Here's how the part is built. I have some questions about the finished solid (model axes, mm). Face numbers are marked on the shaded views. Coordinates: 2 decimals unless noted, no trailing zeros. Write each loop counter-clockwise with the first axis right and the second up, starting at its lowest first coordinate (ties: lowest second). Pieces come first, ordered by that corner, then holes.
Autodesk Inventor part; units mm, degrees
ref_plane "YZ Plane" through (0, 0, 0) normal (1, 0, 0) x (0, 1, 0)
ref_plane "XZ Plane" through (0, 0, 0) normal (0, 1, 0) x (-1, 0, 0)
ref_plane "XY Plane" through (0, 0, 0) normal (0, 0, 1) x (1, 0, 0)
sketch "Sketch1" plane through (0, 0, 0) normal (0, 0, 1) x (1, 0, 0)
  circle A0 centre (0, 0) radius 52.75
  dimension "d0" = 105.5
extrude "Extrusion1" add sketch "Sketch1" along normal blind 7
fillet "Fillet1" radius 4 1 edges at (-52.75, 0, 7)
sketch "Sketch2" plane through (0, 0, 0) normal (0, 0, -1) x (-1, 0, 0)
  circle A0 centre (0, 0) radius 51.8
  circle A1 centre (0, 0) radius 52.75
  circle A2 centre (0, 0) radius 52.75
  dimension "d4" = 103.6
  dimension "d69" = 0
extrude "Extrusion2" cut sketch "Sketch2" against normal blind 3
sketch "Sketch3" plane through (0, 0, 0) normal (0, 0, -1) x (-1, 0, 0)
  circle A0 centre (0, 0) radius 48.75
extrude "Extrusion3" cut sketch "Sketch3" against normal blind 6
sketch "Sketch6" plane through (0, 0, 7) normal (0, 0, 1) x (1, 0, 0)
  circle A0 centre (0, 0) radius 15 construction
  circle A1 centre (15, 0) radius 1
  circle A2 centre (14.0954, 5.1303) radius 1
  circle A3 centre (11.4907, 9.6418) radius 1
  circle A4 centre (7.5, 12.9904) radius 1
  circle A5 centre (2.6047, 14.7721) radius 1
  circle A6 centre (-2.6047, 14.7721) radius 1
  circle A7 centre (-7.5, 12.9904) radius 1
  circle A8 centre (-11.4907, 9.6418) radius 1
  circle A9 centre (-14.0954, 5.1303) radius 1
  circle A10 centre (-15, 0) radius 1
  circle A11 centre (-14.0954, -5.1303) radius 1
  circle A12 centre (-11.4907, -9.6418) radius 1
  circle A13 centre (-7.5, -12.9904) radius 1
  circle A14 centre (-2.6047, -14.7721) radius 1
  circle A15 centre (2.6047, -14.7721) radius 1
  circle A16 centre (7.5, -12.9904) radius 1
  circle A17 centre (11.4907, -9.6418) radius 1
  circle A18 centre (14.0954, -5.1303) radius 1
  circle A19 centre (0, 0) radius 10 construction
  circle A20 centre (0, -10) radius 1
  circle A21 centre (4.3388, -9.0097) radius 1
  circle A22 centre (7.8183, -6.2349) radius 1
  circle A23 centre (9.7493, -2.2252) radius 1
  circle A24 centre (9.7493, 2.2252) radius 1
  circle A25 centre (7.8183, 6.2349) radius 1
  circle A26 centre (4.3388, 9.0097) radius 1
  circle A27 centre (0, 10) radius 1
  circle A28 centre (-4.3388, 9.0097) radius 1
  circle A29 centre (-7.8183, 6.2349) radius 1
  circle A30 centre (-9.7493, 2.2252) radius 1
  circle A31 centre (-9.7493, -2.2252) radius 1
  circle A32 centre (-7.8183, -6.2349) radius 1
  circle A33 centre (-4.3388, -9.0097) radius 1
  circle A34 centre (0, 0) radius 5 construction
  circle A35 centre (0, -5) radius 1
  circle A36 centre (4.3301, -2.5) radius 1
  circle A37 centre (4.3301, 2.5) radius 1
  circle A38 centre (0, 5) radius 1
  circle A39 centre (-4.3301, 2.5) radius 1
  circle A40 centre (-4.3301, -2.5) radius 1
  dimension "d44" = 30
  dimension "d50" = 20
  dimension "d56" = 10
  dimension "d45" = 2
  dimension "d48" = 360
  dimension "d51" = 2
  dimension "d54" = 360
  dimension "d57" = 2
  dimension "d60" = 360
hole "Hole1" at (0, 5, 7) at (0, 10, 7) at (4.3388, 9.0097, 7) at (7.8183, 6.2349, 7) at (7.5, 12.9904, 7) at (4.3301, 2.5, 7) at (9.7493, 2.2252, 7) at (0, 0, 7) at (0, 0, 7) at (0, 0, 7) at (4.3301, -2.5, 7) at (-7.8183, 6.2349, 7) at (-4.3301, -2.5, 7) at (0, -5, 7) at (0, 0, 7) at (15, 0, 7) at (14.0954, 5.1303, 7) at (11.4907, 9.6418, 7) at (2.6047, 14.7721, 7) at (-4.3388, 9.0097, 7) at (-11.4907, 9.6418, 7) at (-7.5, 12.9904, 7) at (-2.6047, 14.7721, 7) at (11.4907, -9.6418, 7) at (9.7493, -2.2252, 7) at (7.8183, -6.2349, 7) at (14.0954, -5.1303, 7) at (-14.0954, 5.1303, 7) at (-15, 0, 7) at (-14.0954, -5.1303, 7) at (-11.4907, -9.6418, 7) at (-7.5, -12.9904, 7) at (-4.3301, 2.5, 7) at (-4.3388, -9.0097, 7) at (-7.8183, -6.2349, 7) at (-9.7493, 2.2252, 7) at (-9.7493, -2.2252, 7) at (-2.6047, -14.7721, 7) at (2.6047, -14.7721, 7) at (7.5, -12.9904, 7) at (4.3388, -9.0097, 7) at (0, -10, 7) direction (0, 0, -1) diameter 1.778 depth 10.688
fillet "Fillet2" radius 2 1 edges at (48.75, 0, 6)
properties part number "lid_top" material "PC/ABS Plastic"
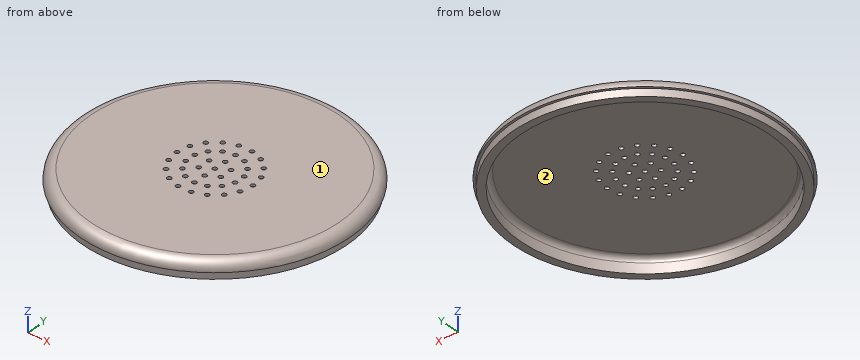
1) Imagine slicing it at A-A on z = 1.25. Please give me the cut outline in (x, y).
Values follow:
outline: circle Ø103.6 at (0, 0); hole circle Ø97.5 at (0, 0)
2) Will these pins go through, and if not, where does the flat tip stop? pin 1 (2 mm diameter, centred on x = -14.1, y = -5.13, fed in from -Z); pin 2 (1.5 mm diameter, centred on x = 30, z = 2, fed in from +Y).
Values follow:
pin 1: stops at z = 6
pin 2: stops at y = 42.75
3) I need wall thicknesses on probe 1 along X at (y, z) = (-5, 6.25); probe 2 along X at (y, z) = (2.5, 6.55); probe 3 along Y at (x, z) = (0, 2.8). Which ranges of each line are inside material? Lowest first, please.
Values follow:
probe 1: x = -50.84 to -14.97, -13.22 to -0.89, 0.89 to 13.22, 14.97 to 50.84
probe 2: x = -50.53 to -10.59, -8.9 to -5.22, -3.44 to 3.44, 5.22 to 8.9, 10.59 to 50.53
probe 3: y = -51.8 to -48.75, 48.75 to 51.8
4) We'd pull the mould along Y, two halves only. Please class the marked faces 1 and 2: pulls with the +Y half, pulls with the -Y half, needs draft (parallel to the pull), parting line crosses it, or undercut.
Values follow:
face 1: needs draft
face 2: undercut
